CAD build for the part. Positions are in the model's coordinates, mm. A direction names the side the tool comes from. Give positions to 0.01 mm unless a question says otherwise; leave off trailing zeros. Write each loop counter-clockwise with the first axis right and the second up, starting at its lowest first coordinate (ties: lowest second). Pieces come first, ordered by that corner, then holes. Notation, with made-up numbers: (35.25, 40) -> (50.25, 40) arc R27 cw to (50.25, 56) -> close; hole circle Ø6 at (14, 72). An arc over 180 degrees is marked (long way). Answer as a JSON object with one key per item and string values.
```python
from build123d import *

# Parameters (mm, degrees)
SKETCH2_R           = 5
BOSS_EXTRUDE1_DEPTH = 6
SKETCH4_R           = 6.5
CUT_EXTRUDE2_DEPTH  = 4


with BuildPart() as part:
    # Sketch2 → Boss-Extrude1 (new body)
    with BuildSketch(Plane(origin=(0, 0, 0), x_dir=(1, 0, 0), z_dir=(0, 1, 0))):
        with BuildLine():
            Line((-45, 15), (350, 15))
            ThreePointArc((350, 15), (365, 0), (350, -15))
            Line((350, -15), (-45, -15))
            ThreePointArc((-45, -15), (-60, 0), (-45, 15))
        make_face()
        with Locations(Location((-45, 0, 0), (0, 0, 270))):
            Circle(SKETCH2_R, mode=Mode.SUBTRACT)
        with Locations(Location((350, 0, 0), (0, 0, 270))):
            Circle(SKETCH2_R, mode=Mode.SUBTRACT)
    extrude(amount=BOSS_EXTRUDE1_DEPTH)

    # Sketch4 → Cut-Extrude2 (cut)
    with BuildSketch(Plane(origin=(0, 6, 0), x_dir=(1, 0, 0), z_dir=(0, 1, 0))):
        with Locations(Location((-45, 0, 0), (0, 0, 270))):
            Circle(SKETCH4_R)
        with Locations(Location((350, 0, 0), (0, 0, 270))):
            Circle(SKETCH4_R)
    extrude(amount=-CUT_EXTRUDE2_DEPTH, mode=Mode.SUBTRACT)


solid = part.part
```
1) Slice it at B-B (y = 3.4). List the corners of the cut face in (x, z), then the cut area to 3 significant figures.
Model answer:
{"outline": "(-45, -15) -> (350, -15) arc R15 ccw to (350, 15) -> (-45, 15) arc R15 ccw to start; hole circle Ø13 at (-45, 0); hole circle Ø13 at (350, 0)", "area": "12,300 mm2"}
2) Pin check, flat tips, straight feed: pin 1 (6.5 mm diameter, centred on x = -42.5, z = -2, fed in from +Y); pin 2 (11.5 mm diameter, centred on x = -45, z = 0, fed in from -Y); pin 3 (4 mm diameter, centred on x = 351.5, z = 0.5, fed in from +Y); pin 4 (3 mm diameter, centred on y = 1, z = -2.5, fed in from -X). Stop position of each tip, or through.
Model answer:
{"pin 1": "stops at y = 2", "pin 2": "stops at y = 0", "pin 3": "passes through", "pin 4": "stops at x = -59.97"}
3) Mould opens along X. For faces 3 (the cylindrical face through (354.957, 0.986, -0.651)), 4 (the flat face through (155, 6, 0)), 5 (the cylindrical face through (365, 3, 0)), 6 (the flat face through (345, 2, 2)) say: released by +X, released by -X, zero draft, split by the parting line, or undercut.
Model answer:
{"face 3": "undercut", "face 4": "zero draft", "face 5": "released by +X", "face 6": "undercut"}
4) Wall check: probe 1 along X at (y, z) = (4.1, 0); probe 2 along X at (y, z) = (1, 0); probe 3 along Z at (x, y) = (-45, 0.4). Give the ranges that are in metal, low to high.
Model answer:
{"probe 1": "x = -60 to -51.5, -38.5 to 343.5, 356.5 to 365", "probe 2": "x = -60 to -50, -40 to 345, 355 to 365", "probe 3": "z = -15 to -5, 5 to 15"}
5) Slice it at A-A (z = 0). List the corners of the cut face in (x, y), then the cut area to 3 significant figures.
Model answer:
{"outline": "(-60, 0) -> (-50, 0) -> (-50, 2) -> (-51.5, 2) -> (-51.5, 6) -> (-60, 6) -> close; (-40, 0) -> (345, 0) -> (345, 2) -> (343.5, 2) -> (343.5, 6) -> (-38.5, 6) -> (-38.5, 2) -> (-40, 2) -> close; (355, 0) -> (365, 0) -> (365, 6) -> (356.5, 6) -> (356.5, 2) -> (355, 2) -> close", "area": "2,410 mm2"}
6) 3-axis set-ups, long thin cutter, end or side, ignore diameter. For faces 1 (the cylindrical face through (-40.043, 0.986, -0.651)), 2 (the flat face through (-50, 2, 2)): which of +Z, -Z, +X, -X, +Y, -Y reach the whole face in a straight line?
Model answer:
{"face 1": "+Y, -Y", "face 2": "+Y"}
